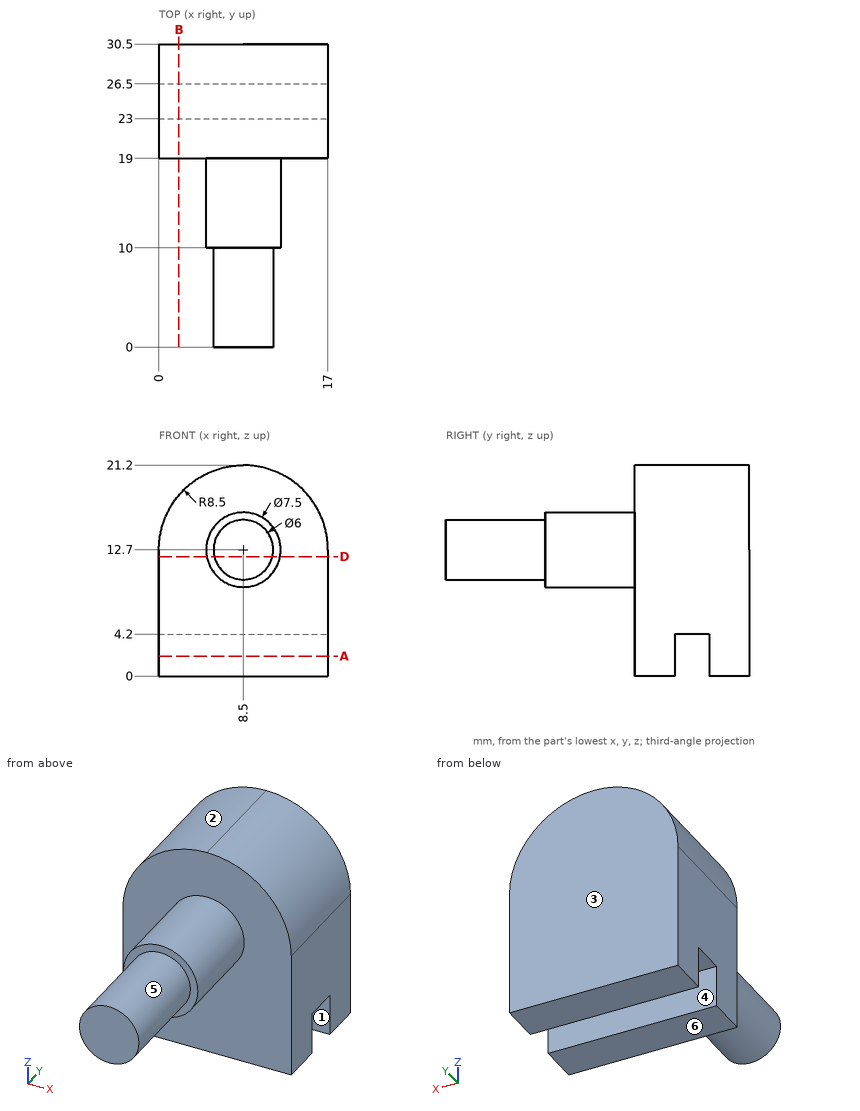
Part print with two shaded views. Sizes in mm from the minimum x, y, z corner. A direction names the side the tool comes from. Round coordinates to 2 decimals unless told otherwise and drop trailing zeros. Order: outer loops, then holes, each group sorted by start corner. A loop starts at its lowest first (then second) coordinate and runs counter-clockwise, first axis right, second up. Notation, with made-up numbers: M 25.25,60 L 82.25,60 A23 cw 82.25,79 Z; hole C -33.5,52 d6. An arc over 180 degrees is marked long. Use CSV: the item, a comma, the result in double quotes.
Item 1: Pin check, flat tips, straight feed: pin 1 (4 mm diameter, centred on x = 9.5, y = 8.5, fed in from +Z); pin 2 (2 mm diameter, centred on x = 5.5, z = 17, fed in from -Y); pin 3 (4 mm diameter, centred on x = 10, y = 9.5, fed in from -Z). Stop position of each tip, or through.
Worked answers:
pin 1,"z = 16.45"
pin 2,"y = 19"
pin 3,"z = 8.95"
Item 2: Probe probe 1 along Y at (x, z) = (9, 3.75); probe 2 along Y at (x, z) = (2, 12.5); probe 3 along Y at (x, z) = (6, 15). List the from-to ranges inside material, lowest first.
Worked answers:
probe 1,"19 to 23, 26.5 to 30.5"
probe 2,"19 to 30.5"
probe 3,"10 to 30.5"
Item 3: Saw through at B-B (x = 2). List the corners of the cut face in (y, z), plus the area to 3 significant figures.
Worked answers:
outline,"M 19,0 L 23,0 L 23,4.2 L 26.5,4.2 L 26.5,0 L 30.5,0 L 30.5,18.18 L 19,18.18 Z"
area,"194 mm²"
Item 4: Pull direction Y, two halves, no side cores. Call the marked faces 1, 2 and 3: released by +Y, released by -Y, zero draft, split by the parting line, or undercut.
Worked answers:
face 1,"undercut"
face 2,"zero draft"
face 3,"released by +Y"
Item 5: Saw through at D-D (z = 12). List the corners of the cut face in (x, y).
Worked answers:
outline,"M 0,19 L 4.82,19 L 4.82,10 L 5.58,10 L 5.58,0 L 11.42,0 L 11.42,10 L 12.18,10 L 12.18,19 L 17,19 L 17,30.5 L 0,30.5 Z"
Item 6: Saw through at A-A (z = 2). List the corners of the cut face in (x, y), plus the area to 3 significant figures.
Worked answers:
outline,"M 0,19 L 17,19 L 17,23 L 0,23 Z; M 0,26.5 L 17,26.5 L 17,30.5 L 0,30.5 Z"
area,"136 mm²"
Item 7: Which spindle directions (+Z, -Z, +X, -X, +Y, -Y) get a long thin tool onto all of the face, cutting with end or side? Do the marked faces 4, 5 and 6. Say none if no direction does.
Worked answers:
face 4,"-Z, +X, -X"
face 5,"-Y"
face 6,"-Z, +X, -X, +Y, -Y"
